Autodesk Inventor part; units mm, degrees
ref_plane "Arbeitsebene1" through (0, 8, 0) normal (0, 1, 0) x (-1, 0, 0)
ref_plane "YZ Plane" through (0, 0, 0) normal (1, 0, 0) x (0, 1, 0)
ref_plane "XY Plane" through (0, 0, 0) normal (0, 0, 1) x (1, 0, 0)
sketch "Skizze1" plane through (0, 0, 0) normal (0, 1, 0) x (-1, 0, 0)
  line L0 (0, 0) -> (10.5, 0)
  line L1 (10.5, 0) -> (10.5, -2)
  line L2 (10.5, -2) -> (8, -2)
  line L3 (8, -2) -> (8, -17)
  line L4 (8, -17) -> (10.5, -17)
  line L5 (10.5, -17) -> (10.5, -19)
  line L6 (10.5, -19) -> (0, -19)
  line L7 (0, -19) -> (0, 0)
  point P0 (0, -9.5)
  dimension "d0" = 2
  dimension "d1" = 2
  dimension "d2" = 21
  dimension "d3" = 16
  dimension "d4" = 19
revolve "Umdrehung1" add sketch "Skizze1" angle 360 about axis through (0, 0, -19) along (0, 0, 1)
sketch "Skizze2" plane through (0, 0, 0) normal (0, 0, 1) x (1, 0, 0)
  circle A0 centre (0, 0) radius 10.5
  point P0 (0, 0)
hole "Bohrung1" at (0, 0, 0) direction (0, 0, -1) diameter 12 end through all
ref_plane "Arbeitsebene1" through (0, 8, 0) normal (0, 1, 0) x (-1, 0, 0)
sketch "Skizze3" plane through (0, 8, 0) normal (0, 1, 0) x (-1, 0, 0)
  line L0 (10.5, 0) -> (-10.5, 0)
  point P0 (0, 0)
  point P1 (0, -9.5)
  point P2 (0, 0)
  dimension "d14" = 9.5
hole "Bohrung2" at (0, 8, -9.5) direction (0, -1, 0) diameter 3 depth 5
equation "\"d1\" = d0"
properties part number "2033" material "Blei"
Geometry check sheet. Reference: the model listing, model coordinates, mm. A direction names the side the tool comes from. Give positions to 0.01 mm unless a question says otherwise; leave off trailing zeros. Order: outer loops, then holes, each group sorted by start corner. A loop starts at its lowest first (then second) coordinate and runs counter-clockwise, first axis right, second up.
1. Sectioned sample at B-B (y = 0). Record the boundary of the cut face in (x, z).
Completed:
outline: (-10.5, -19) - (-6, -19) - (-6, 0) - (-10.5, 0) - (-10.5, -2) - (-8, -2) - (-8, -17) - (-10.5, -17) - close; (6, -19) - (10.5, -19) - (10.5, -17) - (8, -17) - (8, -2) - (10.5, -2) - (10.5, 0) - (6, 0) - close
2. Sectioned sample at D-D (z = -14.25). Record the boundary of the cut face in (x, y), then the cut area to 3 significant figures.
Completed:
outline: circle Ø16 at (0, 0); hole circle Ø12 at (0, 0)
area: 88.0 mm2
3. Scan lines: line 1 (Z direction, x = 8.5, y = 3.25); line 2 (X direction, y = 0, z = -7.5); line 3 (Z direction, x = 0, y = 7.75). Record each from-to range of solid material in increasing order.
Completed:
line 1: z = -19 to -17, -2 to 0
line 2: x = -8 to -6, 6 to 8
line 3: z = -19 to -11, -8 to 0
4. Draft check along X on faces 1 (the face through (-1.802, -5.723, -9.633)), 2 (the face through (-10, 3.2, -1)), 3 (the face through (2, 8, -17)). Enter one of: pulls with the +X half, pulls with the -X half, needs draft (parallel to the pull), parting line crosses it, or undercut.
Completed:
face 1: undercut
face 2: parting line crosses it
face 3: needs draft
5. Sectioned sample at A-A (x = 0). Record the boundary of the cut face in (y, z).
Completed:
outline: (-10.5, -19) - (-6, -19) - (-6, 0) - (-10.5, 0) - (-10.5, -2) - (-8, -2) - (-8, -17) - (-10.5, -17) - close; (6, -19) - (10.5, -19) - (10.5, -17) - (8, -17) - (8, -11) - (6, -11) - close; (6, -8) - (8, -8) - (8, -2) - (10.5, -2) - (10.5, 0) - (6, 0) - close
6. Sectioned sample at C-C (x = 9). Record the boundary of the cut face in (y, z), then the cut area to 3 significant figures.
Completed:
outline: (-5.41, -19) - (5.41, -19) - (5.41, -17) - (-5.41, -17) - close; (-5.41, -2) - (5.41, -2) - (5.41, 0) - (-5.41, 0) - close
area: 43.3 mm2
7. Access from +Z, -Z, +X, -X, +Y, -Y to the whole of each face (thin tool, end or side, straight path). Record for faces 4 (the face through (1.464, 6.889, -9.825)), 5 (the face through (-5, 5, -19)), 6 (the face through (1.73, -7.81, -9.6)).
Completed:
face 4: +Y
face 5: -Z, +X, -X, +Y, -Y
face 6: none
8. Depth check by flat-ended pin: pin 1 (6 mm diameter, centred on x = 1.5, z = -11, fed in from -Y); pin 2 (1 mm diameter, centred on x = -2, z = -3.5, fed in from +Y); pin 3 (5 mm diameter, centred on y = 6, z = -12.5, fed in from +X); pin 4 (11 mm diameter, centred on x = 0, y = 0, fed in from -Z). Enter the tip coordinate at first touch or a pass-through.
Completed:
pin 1: stops at y = -8
pin 2: stops at y = 7.86
pin 3: stops at x = 7.19
pin 4: passes through
